The listing builds one solid part. Answer for the finished solid, in the listing's coordinates (mm). Face numbers are marked on the shaded views. A direction names the side the tool comes from. Round coordinates to 2 decimals unless told otherwise and drop trailing zeros. Write each loop counter-clockwise with the first axis right and the second up, starting at its lowest first coordinate (ties: lowest second). Pieces come first, ordered by that corner, then holes.
(1) A cutting plane is placed at A-A, the plane x = -207. Give the vertices of the cut face in (y, z), and give its area (3 significant figures).
(2) A cutting plane is placed at B-B, the plane z = -10.5. Give the vertices of the cut face in (x, y), and give its area (3 significant figures).
(3) A cutting plane is placed at C-C, the plane y = 95.5. Give the number of separate pieces and of enclosed holes in the cut face, and give its area (3 significant figures).
(4) Find the intervals of material crossed by probe 1 along Y at (x, z) = (-165, -6); probe 2 along X at (y, z) = (79, -13.75); probe 3 along Z at (x, y) = (-166, 82), in increasing order.
(5) Each of these flat-tipped pins is pushed along its axis until it touches: pin 1 Ø3.5 at (x, y) = (-140.46, 79.62) entering from -Z; pin 2 Ø1.6 at (x, y) = (-140.5, 104) entering from +Z; pin 3 Ø7.5 at (x, y) = (-185.5, 95) entering from -Z. Where does it stop, or does it pass through?
(6) For the marked faces 1 and 2, determine the directions among +Z, -Z, +X, -X, +Y, -Y from which every point of the face is accessible in a straight line to the end or side of a thin tool.
(7) The mould has two halves that part along Y. Classify the marked faces 3, 4 and 5: +Y half, -Y half, draft (parallel to the pull), parting line (faces both ways), or undercut.
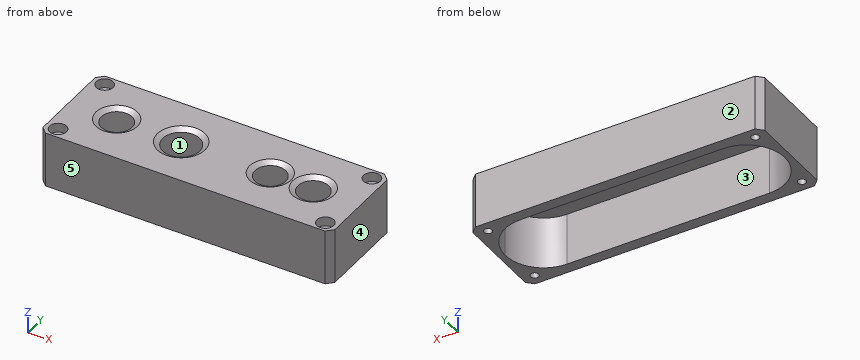
from build123d import *

# Parameters (mm, degrees)
EXTRUDE_1_DEPTH     = 17
SKETCH_2_R          = 6
SKETCH_2_R_2        = 5
EXTRUDE_2_DEPTH     = 1
SKETCH_3_R          = 5
SKETCH_3_R_2        = 6
CUT_EXTRUDE_1_DEPTH = 11
CUT_EXTRUDE_1_TAPER = -60
EXTRUDE_5_DEPTH     = 17
SKETCH_9_R          = 1.3
CUT_EXTRUDE_6_DEPTH = 19.0000001
SKETCH_10_R         = 2.75
CUT_EXTRUDE_7_DEPTH = 3


with BuildPart() as part:
    # 草图1 → 凸台-拉伸1 (new body)
    with BuildSketch(Plane.XY):
        Polygon((-229.462722424, 108.123928313), (-138.462722424, 108.123928313), (-136.462722424, 106.123928313), (-136.462722424, 78.123928313), (-138.462722424, 76.123928313), (-229.462722424, 76.123928313), (-231.462722424, 78.123928313), (-231.462722424, 106.123928313), align=None)
        Polygon((-228.6342953, 106.123928313), (-139.291149549, 106.123928313), (-138.462722424, 105.295501188), (-138.462722424, 78.952355437), (-139.291149549, 78.123928313), (-228.6342953, 78.123928313), (-229.462722424, 78.952355437), (-229.462722424, 105.295501188), align=None, mode=Mode.SUBTRACT)
    extrude(amount=-EXTRUDE_1_DEPTH)

    # 草图2 → 凸台-拉伸2 (add)
    with BuildSketch(Plane.XY):
        Polygon((-136.462722424, 106.123928313), (-138.462722424, 108.123928313), (-229.462722424, 108.123928313), (-231.462722424, 106.123928313), (-231.462722424, 78.123928313), (-229.462722424, 76.123928313), (-138.462722424, 76.123928313), (-136.462722424, 78.123928313), align=None)
        with Locations((-194.962722424, 92.123928313)):
            Circle(SKETCH_2_R, mode=Mode.SUBTRACT)
        with Locations((-165.962722424, 92.123928313)):
            Circle(SKETCH_2_R_2, mode=Mode.SUBTRACT)
        with Locations((-215.962722424, 92.123928313)):
            Circle(SKETCH_2_R_2, mode=Mode.SUBTRACT)
        with Locations((-151.962722424, 92.123928313)):
            Circle(SKETCH_2_R_2, mode=Mode.SUBTRACT)
    extrude(amount=EXTRUDE_2_DEPTH)

    # 草图3 → 切除-拉伸1 (cut)
    with BuildSketch(Plane(origin=(0, 0, 0), x_dir=(-1, 0, 0), z_dir=(0, 0, -1))):
        with Locations((151.962722424, 92.123928313)):
            Circle(SKETCH_3_R)
        with Locations((215.962722424, 92.123928313)):
            Circle(SKETCH_3_R)
        with Locations((194.962722424, 92.123928313)):
            Circle(SKETCH_3_R_2)
        with Locations((165.962722424, 92.123928313)):
            Circle(SKETCH_3_R)
    extrude(amount=-CUT_EXTRUDE_1_DEPTH, taper=CUT_EXTRUDE_1_TAPER, mode=Mode.SUBTRACT)

    # 草图8 → 凸台-拉伸5 (add)
    with BuildSketch(Plane(origin=(0, 0, 0), x_dir=(-1, 0, 0), z_dir=(0, 0, -1))):
        with BuildLine():
            ThreePointArc((229.462722424, 92.123928313), (225.801557189, 83.285093548), (216.962722424, 79.623928313))
            Line((216.962722424, 79.623928313), (150.962722424, 79.623928313))
            ThreePointArc((150.962722424, 79.623928313), (142.123887659, 83.285093548), (138.462722424, 92.123928313))
            Line((138.462722424, 92.123928313), (138.462722424, 78.952355437))
            Line((138.462722424, 78.952355437), (139.291149549, 78.123928313))
            Line((139.291149549, 78.123928313), (228.6342953, 78.123928313))
            Line((228.6342953, 78.123928313), (229.462722424, 78.952355437))
            Line((229.462722424, 78.952355437), (229.462722424, 92.123928313))
        make_face()
        with BuildLine():
            ThreePointArc((216.962722424, 104.623928313), (225.801557189, 100.962763077), (229.462722424, 92.123928313))
            Line((229.462722424, 92.123928313), (229.462722424, 105.295501188))
            Line((229.462722424, 105.295501188), (228.6342953, 106.123928313))
            Line((228.6342953, 106.123928313), (139.291149549, 106.123928313))
            Line((139.291149549, 106.123928313), (138.462722424, 105.295501188))
            Line((138.462722424, 105.295501188), (138.462722424, 92.123928313))
            ThreePointArc((138.462722424, 92.123928313), (142.123887659, 100.962763077), (150.962722424, 104.623928313))
            Line((150.962722424, 104.623928313), (216.962722424, 104.623928313))
        make_face()
    extrude(amount=EXTRUDE_5_DEPTH)

    # 草图9 → 切除-拉伸6 (cut, through all)
    with BuildSketch(Plane(origin=(0, 0, -17), x_dir=(-1, 0, 0), z_dir=(0, 0, -1))):
        with Locations((227.462722424, 79.623928313)):
            Circle(SKETCH_9_R)
        with Locations((227.462722424, 104.623928313)):
            Circle(SKETCH_9_R)
        with Locations((140.462722424, 79.623928313)):
            Circle(SKETCH_9_R)
        with Locations((140.462722424, 104.623928313)):
            Circle(SKETCH_9_R)
    extrude(amount=-CUT_EXTRUDE_6_DEPTH, mode=Mode.SUBTRACT)

    # 草图10 → 切除-拉伸7 (cut)
    with BuildSketch(Plane.XY.offset(1)):
        with Locations((-227.462722424, 104.623928313)):
            Circle(SKETCH_10_R)
        with Locations((-140.462722424, 104.623928313)):
            Circle(SKETCH_10_R)
        with Locations((-227.462722424, 79.623928313)):
            Circle(SKETCH_10_R)
        with Locations((-140.462722424, 79.623928313)):
            Circle(SKETCH_10_R)
    extrude(amount=-CUT_EXTRUDE_7_DEPTH, mode=Mode.SUBTRACT)


solid = part.part
Solutions:
1. outline: (76.12, -17) - (79.62, -17) - (79.62, 0) - (104.62, 0) - (104.62, -17) - (108.12, -17) - (108.12, 1) - (76.12, 1) - close
1. area: 151 mm2
2. outline: (-231.46, 78.12) - (-229.46, 76.12) - (-138.46, 76.12) - (-136.46, 78.12) - (-136.46, 106.12) - (-138.46, 108.12) - (-229.46, 108.12) - (-231.46, 106.12) - close; hole circle Ø2.6 at (-227.46, 79.62); hole circle Ø2.6 at (-227.46, 104.62); hole (-216.96, 79.62) - (-150.96, 79.62) arc R12.5 ccw to (-150.96, 104.62) - (-216.96, 104.62) arc R12.5 ccw to start; hole circle Ø2.6 at (-140.46, 79.62); hole circle Ø2.6 at (-140.46, 104.62)
2. area: 870 mm2
3. separate pieces: 5
3. enclosed holes: 0
3. area: 138 mm2
4. probe 1: y = 76.12 to 79.62, 104.62 to 108.12
4. probe 2: x = -231.46 to -228.6, -226.32 to -141.6, -139.32 to -136.46
4. probe 3: z = 0 to 1
5. pin 1: stops at z = -17
5. pin 2: stops at z = -2
5. pin 3: stops at z = 0
6. face 1: -Z
6. face 2: +Z, -Z, +X, -X, +Y
7. face 3: undercut
7. face 4: draft
7. face 5: -Y half
